Read the model definition and answer for the solid it produces. Units are mm, in the model's axes. Round coordinates to 2 decimals unless told otherwise and drop trailing zeros. Answer as CSV lines item,"result".
```python
from build123d import *

# Parameters (mm, degrees)
F0_W     = 10
F0_H     = 200
F0_R     = 2.5
F1_DEPTH = 6
F2_R     = 4.99999


# Not quite as in the source:
# - a fillet or chamfer is up to 0.001 mm smaller than in the source, because OpenCascade refuses the exact size


with BuildPart() as f1:
    # F0 (on Front) → F1 (new body)
    with BuildSketch(Plane.XZ):
        Rectangle(F0_W, F0_H)
        with Locations((0, -94)):
            Circle(F0_R, mode=Mode.SUBTRACT)
        with Locations((0, 94)):
            Circle(F0_R, mode=Mode.SUBTRACT)
    extrude(amount=F1_DEPTH)

    # F2 (radius 5 in the source; OpenCascade refuses exactly that, so slightly less here)
    f2_edges = [f1.edges().sort_by_distance(p)[0] for p in [
        (-5, -3, 100),
        (5, -3, 100),
        (5, -3, -100),
        (-5, -3, -100),
    ]]
    fillet(f2_edges, radius=F2_R)


solid = f1.part
```
1) Determine the mould class of faces 1 (the cylindrical face through (3, -3, -99)), 2 (the flat face through (-5, -3, -1)), 3 (the cylindrical face through (-0.33, -2.96, 96.48)), 4 (the cylindrical face through (-0.33, -2.96, -91.52)) for opening direction X: released by +X, released by -X, zero draft, split by the parting line, or undercut.
Evaluation:
face 1,"released by +X"
face 2,"released by -X"
face 3,"undercut"
face 4,"undercut"
2) Find section A-A, the plane y = -2.75. Count the separate pieces of the cut face and the enclosed holes in it, then the cut area to 3 significant figures.
Evaluation:
separate pieces,"1"
enclosed holes,"2"
area,"1,940 mm^2"
3) Straight lines are drawn through the part: line 1 (Z direction, x = 2, y = -5.1); line 2 (Z direction, x = 2.25, y = -2.5); line 3 (Z direction, x = -4.5, y = -3.1). For each, find the intervals that lie inside material, in ascending order.
Evaluation:
line 1,"z = -99.58 to -95.5, -92.5 to 92.5, 95.5 to 99.58"
line 2,"z = -99.47 to -95.09, -92.91 to 92.91, 95.09 to 99.47"
line 3,"z = -97.18 to 97.18"
4) Each of these flat-tipped pins is pushed along its axis until it touches: P1, Ø4, axis at x = -1, z = -71.5, coming from the +Y side; P2, Ø2, axis at x = -2.5, y = -4.5, coming from the +Z side. Where does it stop, or does it pass through?
Evaluation:
P1,"stops at y = 0"
P2,"stops at z = 99.77"
